CAD build for the part. Positions are in the model's coordinates, mm. A direction names the side the tool comes from. Give positions to 0.01 mm unless a question says otherwise; leave off trailing zeros. Write each loop counter-clockwise with the first axis right and the second up, starting at its lowest first coordinate (ties: lowest second). Pieces come first, ordered by that corner, then holes. Notation, with made-up numbers: M -16,3.5 L -7,3.5 A11 ccw -7,10.5 Z; hole C -11.75,7.5 d3. An arc over 180 degrees is marked long. One line per question, with ' | ' between items. Start each with the question number.
1. Flat gauge pins, fed straight in: pin 1 (8 mm diameter, centred on x = 3, z = 0, fed in from -Y); pin 2 (4 mm diameter, centred on y = 13.5, z = 10, fed in from -X); pin 3 (0.6 mm diameter, centred on x = -0.5, y = 9, fed in from +Z); pin 4 (4 mm diameter, centred on y = 1.5, z = 19, fed in from -X). Where does each tip first touch, or does it go through?
2. Cut at C-C, the plane x = 2.5. Write the cut outline in (y, z).
3. Cut at A-A, the plane z = -10.5. Write the cut outline in (x, y), then the cut area to 3 significant figures.
4. Cut at D-D, the plane x = 14.5. Write the cut outline in (y, z), then the cut area to 3 significant figures.
5. Pull direction Z, two halves, no side cores. Call faces 5 (the face through (11, 15, -10)), 6 (the face through (2, 2, 25.009)), 7 (the face through (18, 5, 0)): released by +Z, released by -Z, zero draft, split by the parting line, or undercut.
6. Cut at B-B, the plane y = 1.5. Write the cut outline in (x, z), then the cut area to 3 significant figures.
7. Which spindle directions (+Z, -Z, +X, -X, +Y, -Y) get a long thin tool onto all of the face, cutting with end or side? Do faces 1 (the face through (7, 2, 20)), 2 (the face through (0, 9, 0)), 3 (the face through (15.25, 15, 10)), 4 (the face through (13.155, 14.735, 10.728)). Say none if no direction does.
8. Wall check: L1, parallel to Y at x = 13.15, z = -10.5; L2, parallel to Y at x = 15.3, z = 10.5; L3, parallel to X at y = 1.75, z = -13. Give the ranges that are in metal, low to high.
```python
from build123d import *

# Parameters (mm, degrees)
BOSS_EXTRUDE1_DEPTH = 11
SKETCH3_W           = 22
SKETCH3_H           = 3
BOSS_EXTRUDE2_DEPTH = 17.7
BOSS_EXTRUDE3_DEPTH = 5
SKETCH5_R           = 1.75
CUT_EXTRUDE1_DEPTH  = 37.035744466
SKETCH6_W           = 9
SKETCH6_H           = 9
BOSS_EXTRUDE4_DEPTH = 5
SKETCH7_R           = 2.25
CUT_EXTRUDE2_DEPTH  = 38.573063213
FILLET1_R           = 1
SKETCH8_R           = 2.5
CUT_EXTRUDE3_DEPTH  = 0.75
FILLET2_R           = 0.5
SKETCH10_W          = 14
SKETCH10_H          = 7.2
CUT_EXTRUDE4_DEPTH  = 2.5
FILLET3_R           = 0.5


with BuildPart() as part:
    # Sketch1 → Boss-Extrude1 (new, symmetric)
    with BuildSketch(Plane(origin=(0, 0, 0), x_dir=(0, 0, -1), z_dir=(1, 0, 0))):
        Polygon((-13.0089, 0), (13.0089, 0), (13.0089, 10.5), (5.7589, 10.5), (5.7589, 9), (-5.7589, 9), (-5.7589, 10.5), (-13.0089, 10.5), align=None)
    extrude(amount=BOSS_EXTRUDE1_DEPTH, both=True)

    # Sketch3 → Boss-Extrude2 (add)
    with BuildSketch(Plane.XZ):
        with Locations((0, -14.5089)):
            Rectangle(SKETCH3_W, SKETCH3_H)
        with Locations((0, 14.5089)):
            Rectangle(SKETCH3_W, SKETCH3_H)
    extrude(amount=-BOSS_EXTRUDE2_DEPTH)

    # Sketch4 → Boss-Extrude3 (add)
    with BuildSketch(Plane(origin=(11, 0, 0), x_dir=(0, 0, -1), z_dir=(1, 0, 0))):
        Polygon((-8.8, 17.7), (-16.0089, 17.7), (-16.0089, 0), (16.0089, 0), (16.0089, 17.7), align=None)
    extrude(amount=BOSS_EXTRUDE3_DEPTH)

    # Sketch5 → Cut-Extrude1 (cut, through all)
    with BuildSketch(Plane(origin=(16, 0, 0), x_dir=(0, 0, -1), z_dir=(1, 0, 0))):
        with Locations((-10.5, 13)):
            Circle(SKETCH5_R)
        with Locations((10.5, 13)):
            Circle(SKETCH5_R)
    extrude(amount=-CUT_EXTRUDE1_DEPTH, mode=Mode.SUBTRACT)

    # Sketch6 → Boss-Extrude4 (add)
    with BuildSketch(Plane.XZ):
        with Locations((20.5, 0)):
            Rectangle(SKETCH6_W, SKETCH6_H)
        with Locations((2.5, 20.5089)):
            Rectangle(SKETCH6_W, SKETCH6_H)
    extrude(amount=-BOSS_EXTRUDE4_DEPTH)

    # Sketch7 → Cut-Extrude2 (cut, through all)
    with BuildSketch(Plane(origin=(0, 5, 0), x_dir=(1, 0, 0), z_dir=(0, 1, 0))):
        with Locations(Location((20.5, 0, 0), (0, 0, 270))):
            Circle(SKETCH7_R)
        with Locations(Location((2.5, -20.5089, 0), (0, 0, 270))):
            Circle(SKETCH7_R)
    extrude(amount=-CUT_EXTRUDE2_DEPTH, mode=Mode.SUBTRACT)

    # Fillet1
    fillet1_edges = [part.edges().sort_by_distance(p)[0] for p in [
        (0, 10.5, 5.7589),
        (0, 10.5, -5.7589),
        (25, 5, 0),
        (25, 2.5, 4.5),
        (25, 2.5, -4.5),
        (7, 2.5, 25.0089),
        (2.5, 5, 25.0089),
        (-2, 2.5, 25.0089),
    ]]
    fillet(fillet1_edges, radius=FILLET1_R)

    # Sketch8 → Cut-Extrude3 (cut)
    with BuildSketch(Plane(origin=(16, 0, 0), x_dir=(0, 0, -1), z_dir=(1, 0, 0))):
        with Locations((-10.5, 13)):
            Circle(SKETCH8_R)
        with Locations((10.5, 13)):
            Circle(SKETCH8_R)
    extrude(amount=-CUT_EXTRUDE3_DEPTH, mode=Mode.SUBTRACT)

    # Fillet2
    fillet2_edges = [part.edges().sort_by_distance(p)[0] for p in [
        (16, 13, 13),
        (16, 13, -8),
    ]]
    fillet(fillet2_edges, radius=FILLET2_R)

    # Sketch10 → Cut-Extrude4 (cut)
    with BuildSketch(Plane.ZY.offset(-11)):
        with Locations((0, 14.1)):
            Rectangle(SKETCH10_W, SKETCH10_H)
    extrude(amount=-CUT_EXTRUDE4_DEPTH, mode=Mode.SUBTRACT)

    # Fillet3
    fillet3_edges = [part.edges().sort_by_distance(p)[0] for p in [
        (13.5, 14.1, -7),
        (13.5, 14.1, 7),
        (11, 14.1, -7),
        (11, 14.1, 7),
        (11, 14.1, -13.0089),
        (11, 14.1, 13.0089),
    ]]
    fillet(fillet3_edges, radius=FILLET3_R)


solid = part.part
```
Here are the results:
1) pin 1: y = 0 | pin 2: x = 11 | pin 3: z = 16.01 | pin 4: x = -2
2) outline: M 0,-16.01 L 17.7,-16.01 L 17.7,-13.01 L 10.5,-13.01 L 10.5,-6.76 A1 ccw 9.5,-5.76 L 9,-5.76 L 9,5.76 L 9.5,5.76 A1 ccw 10.5,6.76 L 10.5,13.01 L 17.7,13.01 L 17.7,16.01 L 5,16.01 L 5,18.26 L 0,18.26 Z; M 0,22.76 L 5,22.76 L 5,24.01 A1 ccw 4,25.01 L 0,25.01 Z
3) outline: M -11,0 L 16,0 L 16,10 A0.5 ccw 15.5,10.5 L 15.25,10.5 L 15.25,11.25 L 11,11.25 L 11,10.5 L -11,10.5 Z; M 11,14.75 L 15.25,14.75 L 15.25,15.5 L 15.5,15.5 A0.5 ccw 16,16 L 16,17.7 L 11,17.7 Z | area: 301 mm^2
4) outline: M 0,-16.01 L 17.7,-16.01 L 17.7,16.01 L 0,16.01 Z; hole C 13,-10.5 d3.5; hole C 13,10.5 d3.5 | area: 547 mm^2
5) face 5: undercut | face 6: released by +Z | face 7: zero draft
6) outline: M -11,-16.01 L 16,-16.01 L 16,-4.5 L 24,-4.5 A1 ccw 25,-3.5 L 25,3.5 A1 ccw 24,4.5 L 16,4.5 L 16,16.01 L 7,16.01 L 7,24.01 A1 ccw 6,25.01 L -1,25.01 A1 ccw -2,24.01 L -2,16.01 L -11,16.01 Z; hole C 2.5,20.51 d4.5; hole C 20.5,0 d4.5 | area: 994 mm^2
7) face 1: +Z, +X, +Y, -Y | face 2: -X, +Y | face 3: +X | face 4: +X, -X
8) L1: 0 to 11.25, 14.75 to 17.7 | L2: 0 to 10.5, 15.5 to 17.7 | L3: -11 to 16
